```python
from build123d import *

# Parameters (mm, degrees)
SKETCH1_W           = 100
SKETCH1_H           = 100
BOSS_EXTRUDE1_DEPTH = 50
SKETCH2_R           = 21
CUT_EXTRUDE1_DEPTH  = 87.602540378
SKETCH3_W           = 70
SKETCH3_H           = 50
BOSS_EXTRUDE2_DEPTH = 100
SKETCH4_W           = 100
SKETCH4_H           = 1
CUT_EXTRUDE2_DEPTH  = 213.132034356
SKETCH6_W           = 20
SKETCH6_H           = 10
CUT_EXTRUDE3_DEPTH  = 25
SKETCH7_W           = 10
SKETCH7_H           = 20
CUT_EXTRUDE4_DEPTH  = 10
SKETCH8_W           = 15
SKETCH8_H           = 49
CUT_EXTRUDE5_DEPTH  = 123.069652248
SKETCH9_W           = 14.755371785
SKETCH9_H           = 70
CUT_EXTRUDE6_DEPTH  = 162.635392164
SKETCH10_W          = 10
SKETCH10_H          = 49
CUT_EXTRUDE7_DEPTH  = 195.785965312


with BuildPart() as part:
    # Sketch1 → Boss-Extrude1 (new body)
    with BuildSketch(Plane(origin=(0, 0, 0), x_dir=(1, 0, 0), z_dir=(0, 1, 0))):
        Rectangle(SKETCH1_W, SKETCH1_H)
    extrude(amount=BOSS_EXTRUDE1_DEPTH)

    # Sketch2 → Cut-Extrude1 (cut, through all)
    with BuildSketch(Plane(origin=(0, 50, 0), x_dir=(1, 0, 0), z_dir=(0, 1, 0))):
        with Locations(Location((0, 0, 0), (0, 0, 270))):
            Circle(SKETCH2_R)
    extrude(amount=-CUT_EXTRUDE1_DEPTH, mode=Mode.SUBTRACT)

    # Sketch3 → Boss-Extrude2 (add)
    with BuildSketch(Plane(origin=(50, 0, 0), x_dir=(0, 0, -1), z_dir=(1, 0, 0))):
        with Locations((0, 25)):
            Rectangle(SKETCH3_W, SKETCH3_H)
    extrude(amount=BOSS_EXTRUDE2_DEPTH)

    # Sketch4 → Cut-Extrude2 (cut, through all)
    with BuildSketch(Plane.ZY.offset(50)):
        with Locations((0, 49.5)):
            Rectangle(SKETCH4_W, SKETCH4_H)
    extrude(amount=-CUT_EXTRUDE2_DEPTH, mode=Mode.SUBTRACT)

    # Sketch6 → Cut-Extrude3 (cut)
    with BuildSketch(Plane(origin=(150, 0, 0), x_dir=(0, 0, -1), z_dir=(1, 0, 0))):
        with Locations((0, 5)):
            Rectangle(SKETCH6_W, SKETCH6_H)
    extrude(amount=-CUT_EXTRUDE3_DEPTH, mode=Mode.SUBTRACT)

    # Sketch7 → Cut-Extrude4 (cut)
    with BuildSketch(Plane.XZ.offset(-10)):
        with Locations((130, 0)):
            Rectangle(SKETCH7_W, SKETCH7_H)
    extrude(amount=-CUT_EXTRUDE4_DEPTH, mode=Mode.SUBTRACT)

    # Sketch8 → Cut-Extrude5 (cut, through all)
    with BuildSketch(Plane(origin=(50, 0, 0), x_dir=(0, 0, -1), z_dir=(1, 0, 0))):
        with Locations((42.5, 24.5)):
            Rectangle(SKETCH8_W, SKETCH8_H)
        with Locations((-42.5, 24.5)):
            Rectangle(SKETCH8_W, SKETCH8_H)
    extrude(amount=-CUT_EXTRUDE5_DEPTH, mode=Mode.SUBTRACT)

    # Sketch9 → Cut-Extrude6 (cut, through all)
    with BuildSketch(Plane(origin=(0, 49, 0), x_dir=(1, 0, 0), z_dir=(0, 1, 0))):
        with Locations((-42.622314108, 0)):
            Rectangle(SKETCH9_W, SKETCH9_H)
    extrude(amount=-CUT_EXTRUDE6_DEPTH, mode=Mode.SUBTRACT)

    # Sketch10 → Cut-Extrude7 (cut, through all)
    with BuildSketch(Plane.ZY.offset(35.244628215)):
        with Locations((-30, 24.5)):
            Rectangle(SKETCH10_W, SKETCH10_H)
        with Locations((30, 24.5)):
            Rectangle(SKETCH10_W, SKETCH10_H)
    extrude(amount=-CUT_EXTRUDE7_DEPTH, mode=Mode.SUBTRACT)


solid = part.part
```
Input: part model. Units: mm. Frame: model coordinates. A direction names the side the tool comes from. Give positions to 0.01 mm unless a question says otherwise; leave off trailing zeros. Write each loop counter-clockwise with the first axis right and the second up, starting at its lowest first coordinate (ties: lowest second). Pieces come first, ordered by that corner, then holes. Notation, with made-up numbers: (-12, 49.5) - (10, 49.5) arc R14 ccw to (10, 67.5) - close; hole circle Ø1 at (-14.75, 4). An arc over 180 degrees is marked (long way). Write item = value, one per line. Start each with the question number.
1) Pin query (flat end, axial travel): pin 1 (4.5 mm diameter, centred on x = 145.5, z = -4, fed in from -Y). Return the tip coordinate at first contact, or that it passes through.
2) Cut plane C-C (x = 0). Return loops of the section in (y, z).
3) Material intervals for L1, parallel to X at y = 32.5, z = 0; L2, parallel to X at y = 13.5, z = 7; L3, parallel to Z at x = -12, y = 23, sorted ascending. Write a range as [from, to].
4) Draft query along X for faces 1 (the face through (56, 24, 25)), 2 (the face through (-35.245, 25, 0)), 3 (the face through (135, 15, 0)). Return one class per face: pulls with the +X half, pulls with the -X half, needs draft (parallel to the pull), parting line crosses it, or undercut.
5) Reachability of faces 4 (the face through (130, 20, 0)), 5 (the face through (143, 10, 0)), 6 (the face through (56, 0, 0)) from +Z, -Z, +X, -X, +Y, -Y: full face, straight path, thin tool, end or side. Return the list, or none.
6) Cut plane A-A (z = 0). Return loops of the section in (x, y).
7) Cut plane B-B (y = 16.5). Return loops of the section in (x, z).
8) Cut plane D-D (y = 37). Return loops of the section in (x, z), and give its area (3 significant figures).
Answers follow:
q1.pin_1 = 10
q2.outline = (0, -25) - (49, -25) - (49, -21) - (0, -21) - close; (0, 21) - (49, 21) - (49, 25) - (0, 25) - close
q3.L1 = [-35.24, -21], [21, 150]
q3.L2 = [-35.24, -19.8], [19.8, 125], [135, 150]
q3.L3 = [-25, -17.23], [17.23, 25]
q4.face_1 = needs draft
q4.face_2 = pulls with the -X half
q4.face_3 = undercut
q5.face_4 = -Y
q5.face_5 = +X, -Y
q5.face_6 = +Z, -Z, +X, -X, -Y
q6.outline = (-35.24, 0) - (-21, 0) - (-21, 49) - (-35.24, 49) - close; (21, 0) - (125, 0) - (125, 20) - (135, 20) - (135, 10) - (150, 10) - (150, 49) - (21, 49) - close
q7.outline = (-35.24, -25) - (150, -25) - (150, 25) - (-35.24, 25) - close; hole circle Ø42 at (0, 0); hole (125, -10) - (135, -10) - (135, 10) - (125, 10) - close
q8.outline = (-35.24, -25) - (150, -25) - (150, 25) - (-35.24, 25) - close; hole circle Ø42 at (0, 0)
q8.area = 7,880 mm^2
